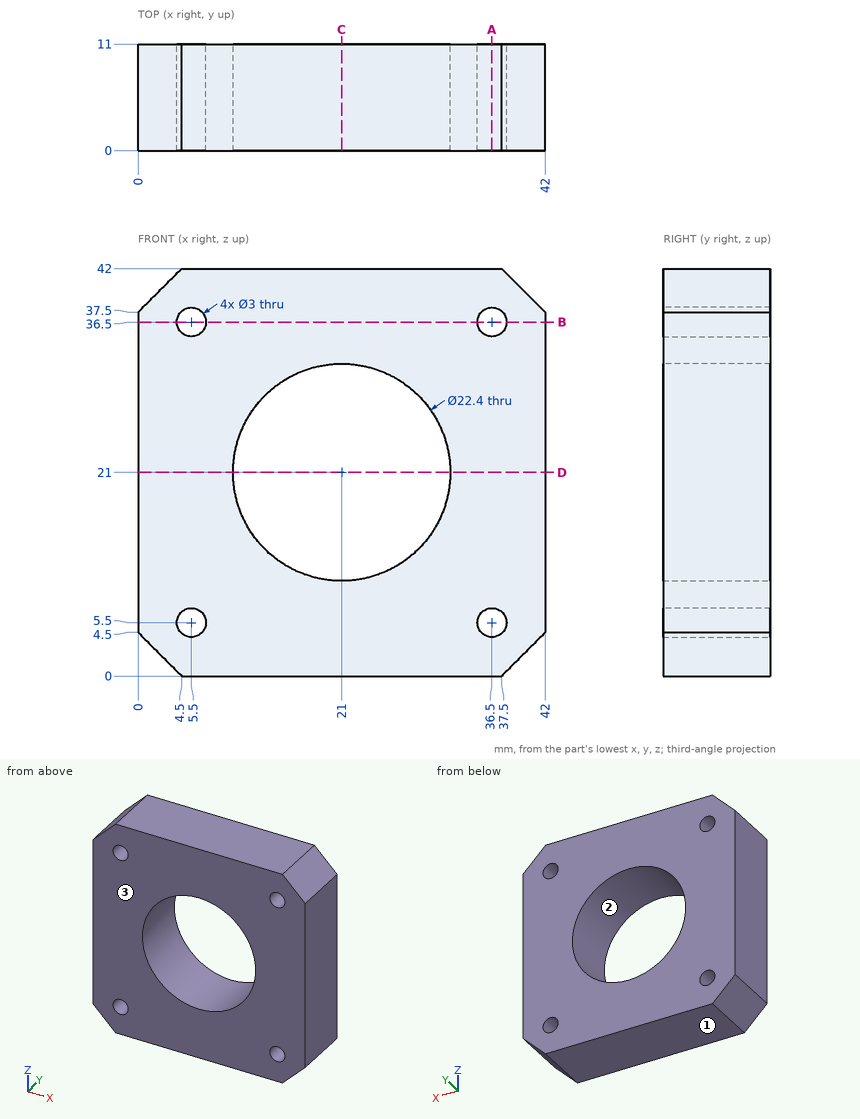
Print and shaded views of the part. All mm, measured from the part's lowest x, y and z. Round coordinates to 2 decimals unless told otherwise and drop trailing zeros. Write each loop counter-clockwise with the first axis right and the second up, starting at its lowest first coordinate (ties: lowest second). Pieces come first, ordered by that corner, then holes. Notation, with made-up numbers: M 24.5,89 L 65.5,89 A9 ccw 65.5,100 Z; hole C -27,-39 d6. An arc over 180 degrees is marked long. Use a Markdown table: item, result. Add a question column.
1. Drill centre lines: probe 1 along X at (y, z) = (2.5, 36.5); probe 2 along Z at (x, y) = (37.5, 5); probe 3 along Z at (x, y) = (29.5, 2). Where is each one in solid material? Low to high.
2. Slice it at D-D on z = 21. Give the cut face in (x, y), then the cut area to 3 significant figures.
3. Pull direction Z, two halves, no side cores. Call the marked faces 1, 2 and 3: released by +Z, released by -Z, zero draft, split by the parting line, or undercut.
4. Slice it at A-A on x = 36.5. Give the cut face in (y, z), then the cut area to 3 significant figures.
5. Slice it at C-C on x = 21. Give the cut face in (y, z), then the cut area to 3 significant figures.
6. Slice it at B-B on z = 36.5. Give the cut face in (x, y), then the cut area to 3 significant figures.
Reply:
| question | item | result |
|---|---|---|
| 1 | probe 1 | x = 0 to 4, 7 to 35, 38 to 42 |
| 1 | probe 2 | z = 0 to 4.38, 6.62 to 35.38, 37.62 to 42 |
| 1 | probe 3 | z = 0 to 13.71, 28.29 to 42 |
| 2 | outline | M 0,0 L 9.8,0 L 9.8,11 L 0,11 Z; M 32.2,0 L 42,0 L 42,11 L 32.2,11 Z |
| 2 | area | 216 mm^2 |
| 3 | face 1 | released by -Z |
| 3 | face 2 | undercut |
| 3 | face 3 | zero draft |
| 4 | outline | M 0,0 L 11,0 L 11,4 L 0,4 Z; M 0,7 L 11,7 L 11,35 L 0,35 Z; M 0,38 L 11,38 L 11,42 L 0,42 Z |
| 4 | area | 396 mm^2 |
| 5 | outline | M 0,0 L 11,0 L 11,9.8 L 0,9.8 Z; M 0,32.2 L 11,32.2 L 11,42 L 0,42 Z |
| 5 | area | 216 mm^2 |
| 6 | outline | M 0,0 L 4,0 L 4,11 L 0,11 Z; M 7,0 L 35,0 L 35,11 L 7,11 Z; M 38,0 L 42,0 L 42,11 L 38,11 Z |
| 6 | area | 396 mm^2 |
